from build123d import *

# Parameters (mm, degrees)
BOSS_EXTRUDE1_DEPTH  = 1.5625
MIRROR4_COPY_1_DEPTH = 1.5625
FILLET1_R            = 5
CUT_EXTRUDE1_START   = -4.125
CUT_EXTRUDE1_DEPTH   = 5.125


with BuildPart() as part:
    # Sketch1 → Boss-Extrude1 (new body, symmetric)
    with BuildSketch(Plane(origin=(0, 0, 0), x_dir=(1, 0, 0), z_dir=(0, 1, 0))):
        Polygon((0, 41), (35, 41), (35, 31.5), (28.5, 31.5), (28.5, 33.5), (26, 33.5), (26, 31.5), (24, 31.5), (24, 28.5), (26, 28.5), (26, 26.5), (28.5, 26.5), (28.5, 28.5), (35, 28.5), (35, 0), (0, 0), align=None)
    boss_extrude1 = extrude(amount=BOSS_EXTRUDE1_DEPTH, both=True)

    # Mirror1: Boss-Extrude1 across plane
    add(boss_extrude1.mirror(Plane(origin=(0, 0, 0), x_dir=(0, 0, 1), z_dir=(1, 0, 0))))

    # Mirror4: Boss-Extrude1 across plane
    add(boss_extrude1.mirror(Plane.XY))

    # Mirror4 copy 1 sketch → Mirror4 copy 1 (add, symmetric)
    with BuildSketch(Plane(origin=(0, 0, 0), x_dir=(-1, 0, 0), z_dir=(0, 1, 0))):
        Polygon((0, 41), (35, 41), (35, 31.5), (28.5, 31.5), (28.5, 33.5), (26, 33.5), (26, 31.5), (24, 31.5), (24, 28.5), (26, 28.5), (26, 26.5), (28.5, 26.5), (28.5, 28.5), (35, 28.5), (35, 0), (0, 0), align=None)
    extrude(amount=MIRROR4_COPY_1_DEPTH, both=True)

    # Fillet1
    fillet1_edges = [part.edges().sort_by_distance(p)[0] for p in [
        (35, 0, 41),
        (35, 0, -41),
        (-35, 0, -41),
        (-35, 0, 41),
    ]]
    fillet(fillet1_edges, radius=FILLET1_R)

    # Sketch2 → Cut-Extrude1 (cut)
    with BuildSketch(Plane(origin=(0, 1.5625, 0), x_dir=(1, 0, 0), z_dir=(0, 1, 0)).offset(CUT_EXTRUDE1_START)):
        Polygon((0, 22.5), (0, -22.5), (-10, -22.5), (-10, 0), (-20, 0), align=None)
    cut_extrude1 = extrude(amount=CUT_EXTRUDE1_DEPTH, mode=Mode.SUBTRACT)

    # Mirror5: Cut-Extrude1 across plane
    add(cut_extrude1.mirror(Plane(origin=(0, 0, 0), x_dir=(0, 0, 1), z_dir=(1, 0, 0))), mode=Mode.SUBTRACT)


solid = part.part
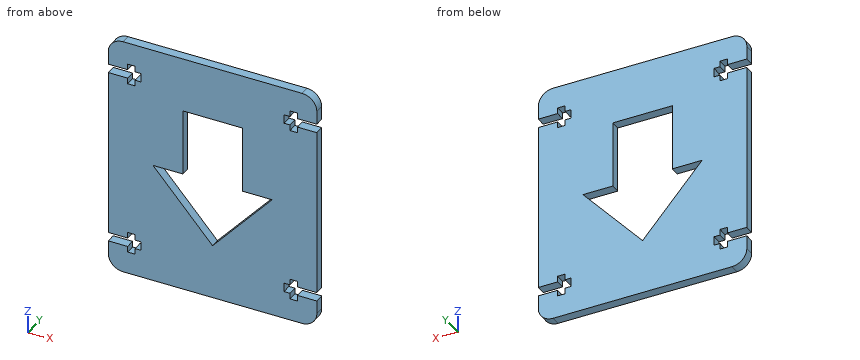
The model under review builds one solid part; all positions refer to its coordinate system, in mm. Give positions to 0.01 mm unless a question says otherwise; leave off trailing zeros. Loops run counter-clockwise (first coordinate to the right, second up) from the corner with the lowest first, then second, coordinate; pieces in that order, holes last. Notation, with made-up numbers: (-20.5, -33) -> (6.5, -33) arc R22 ccw to (6.5, -12) -> close; hole circle Ø9 at (51.25, 73). An arc over 180 degrees is marked (long way). Answer as a JSON object with one key per item and string values. Group by question number.
Q1. Wall thickness on line 1 along X through (y, z) = (1.45, 5.5); line 2 along Z through (x, y) = (0, 0.2); line 3 along X through (y, z) = (0.1, -18): over which ranges is each line inside the solid? List them lowest first.
Q2. Take a section at B-B (z = 17). Write out the cut boundary in (x, y), plus the area to 3 significant figures.
Q3. Take a section at A-A (x = 8). Write out the cut boundary in (y, z), plus the area to 3 significant figures.
Q4. Insertion check: pin 1 (0.9 mm diameter, centred on y = 0, z = 30, fed in from -X); pin 2 (1.6 mm diameter, centred on x = -31, y = -0.5, fed in from +Z). Each pin has a flat end and moves straight along its axis. Give the tip position at first contact, or say it passes through.
Answer below:
{
 "1": {"line 1": "x = -35 to -10, 10 to 35", "line 2": "z = -41 to -22.5, 22.5 to 41", "line 3": "x = -35 to -4, 4 to 35"},
 "2": {"outline": "(-35, -1.56) -> (-10, -1.56) -> (-10, 1.56) -> (-35, 1.56) -> close; (10, -1.56) -> (35, -1.56) -> (35, 1.56) -> (10, 1.56) -> close", "area": "156 mm2"},
 "3": {"outline": "(-1.56, -41) -> (1.56, -41) -> (1.56, -13.5) -> (-1.56, -13.5) -> close; (-1.56, 22.5) -> (1.56, 22.5) -> (1.56, 41) -> (-1.56, 41) -> close", "area": "144 mm2"},
 "4": {"pin 1": "stops at x = -24", "pin 2": "stops at z = 41"}
}
